Read the model definition and answer for the solid it produces. Units are mm, in the model's axes. Face numbers are marked on the shaded views. A direction names the side the tool comes from. Coordinates: 2 decimals unless noted, no trailing zeros. Write each loop counter-clockwise with the first axis right and the second up, starting at its lowest first coordinate (ties: lowest second). Pieces come first, ordered by that corner, then holes.
(1) Section B-B on y = 0 is taken. Write down the section's boundary in (x, z).
(2) Given pin 1 (5 mm diameter, centred on x = 0, z = 10, fed in from +Y); pin 2 (9 mm diameter, centred on x = 0.5, z = 10.5, fed in from +Y); pin 3 (6 mm diameter, centred on x = 0, z = 10, fed in from -Y), each flat-ended and moving along its own axis, determine where each tip first touches the part or whether it passes through.
(3) Section A-A on x = 0 is taken. Write down the section's boundary in (y, z).
(4) Which of the six approach directions +Z, -Z, +X, -X, +Y, -Y give full straight-line access (tool end or side, diameter ignored) to the marked faces 1, 2 and 3?
(5) Section C-C on z = 10 is taken. State how many separate pieces and enclosed holes the cut face has, then the cut area to 3 significant figures.
(6) The mould has two halves that part along X. Classify the marked faces 4, 5, 6 and 7: +X half, -X half, draft (parallel to the pull), parting line (faces both ways), or undercut.
(7) Find the intervals of material crossed by probe 1 along Y at (x, z) = (16.5, 13); probe 2 along X at (y, z) = (4.95, 10); probe 3 along X at (y, z) = (8, 3), in increasing order.
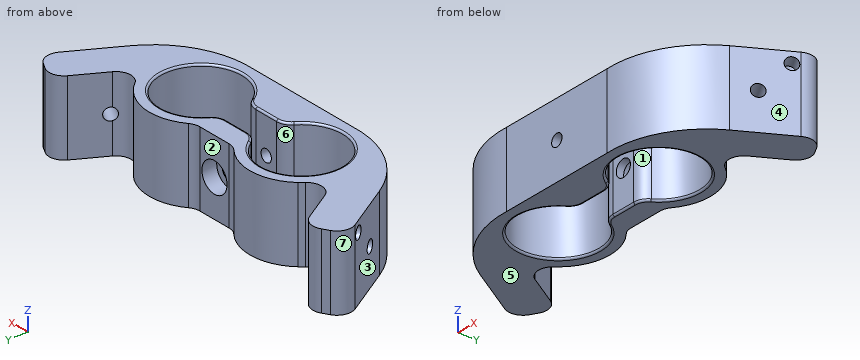
from build123d import *

# Parameters (mm, degrees)
EXTRUDE_2_DEPTH             = 20
HOLE_WIZARD_M41_D           = 4.5
HOLE_WIZARD_M41_DEPTH       = 6
HOLE_WIZARD_M41_CBORE_D     = 8
HOLE_WIZARD_M41_CBORE_DEPTH = 4
M4X0_71_D                   = 3.3
EXTRUDE_4_DEPTH             = 20
CUT_EXTRUDE_1_DEPTH         = 21
FILLET_1_R                  = 4
M4X0_72_D                   = 3.3
FILLET_6_R                  = 0.5


with BuildPart() as part:
    # Эскиз1 → Бобышка-Вытянуть2 (new body)
    with BuildSketch(Plane.XY):
        with BuildLine():
            Line((-6.202041029, 10), (6.202041029, 10))
            ThreePointArc((6.202041029, 10), (16.267083523, 13.997452139), (26.172305548, 9.618950039))
            Line((26.172305548, 9.618950039), (34.464101615, 23.980762114))
            Line((34.464101615, 23.980762114), (43.124355653, 18.980762114))
            Line((43.124355653, 18.980762114), (28.124355653, -7))
            ThreePointArc((28.124355653, -7), (23, -12.124355653), (16, -14))
            Line((16, -14), (-16, -14))
            ThreePointArc((-16, -14), (-23, -12.124355653), (-28.124355653, -7))
            Line((-28.124355653, -7), (-43.124355653, 18.980762114))
            Line((-43.124355653, 18.980762114), (-34.464101615, 23.980762114))
            Line((-34.464101615, 23.980762114), (-26.172305548, 9.618950039))
            ThreePointArc((-26.172305548, 9.618950039), (-16.267083523, 13.997452139), (-6.202041029, 10))
        make_face()
        with BuildLine():
            Line((-5.753049234, 4), (5.753049234, 4))
            ThreePointArc((5.753049234, 4), (27, 0), (5.753049234, -4))
            Line((5.753049234, -4), (-5.753049234, -4))
            ThreePointArc((-5.753049234, -4), (-27, 0), (-5.753049234, 4))
        make_face(mode=Mode.SUBTRACT)
    extrude(amount=EXTRUDE_2_DEPTH)

    # Цековка для винта с внутренним шестигранником M41
    with Locations(Plane(origin=(0, 10, 0), x_dir=(1, 0, 0), z_dir=(0, 1, 0))):
        with Locations((0, -10)):
            CounterBoreHole(HOLE_WIZARD_M41_D / 2, HOLE_WIZARD_M41_CBORE_D / 2, HOLE_WIZARD_M41_CBORE_DEPTH, depth=HOLE_WIZARD_M41_DEPTH)

    # Отверстие обработанное метчиком M4x0.71 (through all)
    with Locations(Plane(origin=(0, -4, 0), x_dir=(1, 0, 0), z_dir=(0, 1, 0))):
        with Locations((0, -10)):
            Hole(M4X0_71_D / 2)

    # Эскиз15 → Бобышка-Вытянуть4 (add)
    with BuildSketch(Plane.XY.offset(20)):
        with BuildLine():
            Line((43.124355653, 18.980762114), (49.186533479, 15.480762114))
            Line((49.186533479, 15.480762114), (39.679655511, -0.98563355))
            ThreePointArc((39.679655511, -0.98563355), (29.657079347, -10.799308246), (16, -14))
            ThreePointArc((16, -14), (23, -12.124355653), (28.124355653, -7))
            Line((28.124355653, -7), (43.124355653, 18.980762114))
        make_face()
        with BuildLine():
            Line((-49.186533479, 15.480762114), (-39.679655511, -0.98563355))
            ThreePointArc((-39.679655511, -0.98563355), (-29.657079347, -10.799308246), (-16, -14))
            ThreePointArc((-16, -14), (-23, -12.124355653), (-28.124355653, -7))
            Line((-28.124355653, -7), (-43.124355653, 18.980762114))
            Line((-43.124355653, 18.980762114), (-49.186533479, 15.480762114))
        make_face()
    extrude(amount=-EXTRUDE_4_DEPTH)

    # Эскиз16 → Вырез-Вытянуть1 (cut, through all)
    with BuildSketch(Plane.XY.offset(20)):
        with BuildLine():
            Line((40.526279442, 20.480762114), (29.856406461, 2))
            ThreePointArc((29.856406461, 2), (28.603842673, 6.094518019), (26.172305548, 9.618950039))
            Line((26.172305548, 9.618950039), (34.464101615, 23.980762114))
            Line((34.464101615, 23.980762114), (40.526279442, 20.480762114))
        make_face()
        with BuildLine():
            Line((-40.526279442, 20.480762114), (-34.464101615, 23.980762114))
            Line((-34.464101615, 23.980762114), (-26.172305548, 9.618950039))
            ThreePointArc((-26.172305548, 9.618950039), (-28.603842673, 6.094518019), (-29.856406461, 2))
            Line((-29.856406461, 2), (-40.526279442, 20.480762114))
        make_face()
    extrude(amount=-CUT_EXTRUDE_1_DEPTH, mode=Mode.SUBTRACT)

    # Скругление1
    fillet_1_edges = [part.edges().sort_by_distance(p)[0] for p in [
        (-29.856406461, 2, 10),
        (-40.526279442, 20.480762114, 10),
        (-6.202041029, 10, 10),
        (6.202041029, 10, 10),
        (-5.753049234, 4, 10),
        (-5.753049234, -4, 10),
        (5.753049234, -4, 10),
        (5.753049234, 4, 10),
        (49.186533479, 15.480762114, 10),
        (-49.186533479, 15.480762114, 10),
        (40.526279442, 20.480762114, 10),
        (29.856406461, 2, 10),
    ]]
    fillet(fillet_1_edges, radius=FILLET_1_R)

    # Отверстие обработанное метчиком M4x0.72 (through all)
    with Locations(Plane(origin=(31.110785953, -15.827350987, 5.43331307), x_dir=(-0.5, -0.866025404, 0), z_dir=(0.866025404, -0.5, 0))):
        with Locations((-23.151495053, -4.56668693)):
            m4x0_72 = Hole(M4X0_72_D / 2)

    # Зеркальное отражение1: Отверстие обработанное метчиком M4x0.72 across plane
    add(m4x0_72.mirror(Plane.ZY), mode=Mode.SUBTRACT)

    # Эскиз13 → Отверстие обработанное метчиком M4x0.73 (revolve, cut)
    with BuildSketch(Plane(origin=(-46.222067385, 10.346156221, 17.071067812), x_dir=(0.5, -0.866025404, 0), z_dir=(0, 0, 1))):
        Polygon((0, 0), (0, 4.991420021), (1.65, 4), (1.65, 0), align=None)
    m4x0_73 = revolve(axis=Axis((-51.721328699, 7.171156221, 17.071067812), (0.866025404, 0.5, 0)), mode=Mode.SUBTRACT)

    # Зеркальное отражение3: Отверстие обработанное метчиком M4x0.73 across plane
    add(m4x0_73.mirror(Plane.ZY), mode=Mode.SUBTRACT)

    # Скругление6
    fillet_6_edges = [part.edges().sort_by_distance(p)[0] for p in [
        (0, -4, 20),
        (-27, 0, 20),
        (0, 4, 20),
        (27, 0, 20),
        (-5.243606026, 4.497619857, 20),
        (5.243606026, 4.497619857, 20),
        (5.243606026, -4.497619857, 20),
        (-5.243606026, -4.497619857, 20),
        (-27, 0, 0),
        (0, -4, 0),
        (27, 0, 0),
        (0, 4, 0),
        (-5.243606026, 4.497619857, 0),
        (5.243606026, 4.497619857, 0),
        (5.243606026, -4.497619857, 0),
        (-5.243606026, -4.497619857, 0),
    ]]
    fillet(fillet_6_edges, radius=FILLET_6_R)


solid = part.part
Response:
1. outline: (-40.25, 0) - (-27.5, 0) arc R0.5 ccw to (-27, 0.5) - (-27, 19.5) arc R0.5 ccw to (-27.5, 20) - (-40.25, 20) - close; (27, 0.5) arc R0.5 ccw to (27.5, 0) - (40.25, 0) - (40.25, 20) - (27.5, 20) arc R0.5 ccw to (27, 19.5) - close
2. pin 1: stops at y = 6
2. pin 2: stops at y = 10.01
2. pin 3: stops at y = -14
3. outline: (-14, 0) - (-4.5, 0) arc R0.5 ccw to (-4, 0.5) - (-4, 8.35) - (-14, 8.35) - close; (-14, 11.65) - (-4, 11.65) - (-4, 19.5) arc R0.5 ccw to (-4.5, 20) - (-14, 20) - close; (4, 0.5) arc R0.5 ccw to (4.5, 0) - (10, 0) - (10, 6) - (6, 6) - (6, 7.75) - (4, 7.75) - close; (4, 12.25) - (6, 12.25) - (6, 14) - (10, 14) - (10, 20) - (4.5, 20) arc R0.5 ccw to (4, 19.5) - close
4. face 1: +Z, -Z
4. face 2: +Z, -Z, +Y
4. face 3: +Z, -Z, -X, -Y
5. separate pieces: 4
5. enclosed holes: 0
5. area: 1,060 mm2
6. face 4: +X half
6. face 5: draft
6. face 6: undercut
6. face 7: -X half
7. probe 1: y = -14.02 to -10.99, 10.99 to 13.99
7. probe 2: x = -38.13 to -25.82, -5.9 to -2.25, 2.25 to 5.9, 25.82 to 38.13
7. probe 3: x = -44.87 to -33.15, -27.56 to -23.55, -8.45 to 8.45, 23.55 to 27.56, 33.15 to 44.87
